Study the drawing (mm; zero at the part's minimum x, y, z) and answer. Give positions to 0.01 mm unless a question says otherwise; leave off trailing zeros. Order: outer loops, then holes, each group sorted by start corner. A loop starts at its lowest first (then second) coordinate and runs counter-clockwise, first axis right, second up. Notation, with made-up numbers: (70.5, 19) - (104.5, 19) arc R23 cw to (104.5, 35) - close; hole circle Ø8 at (11.5, 51). An arc over 180 degrees is marked (long way). Use CSV: the item, a comma, the result in double quotes.
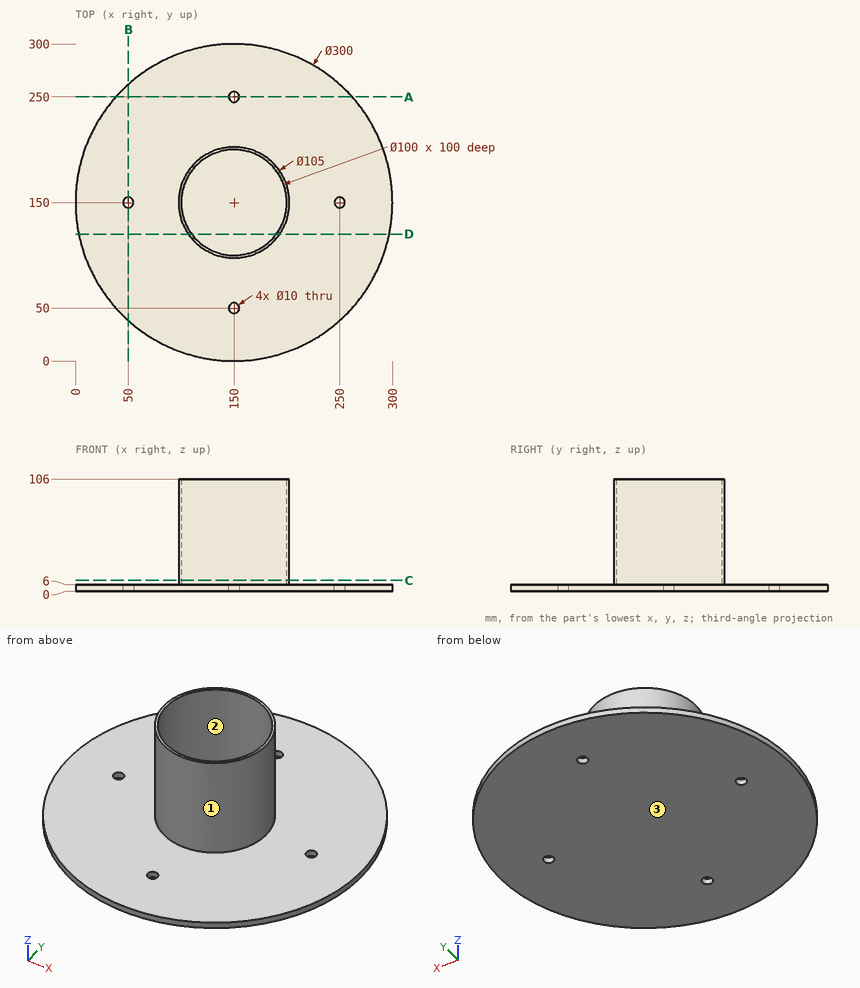
Item 1: The mould has two halves that part along Y. Classify the marked faces 1, 2 and 3: +Y half, -Y half, draft (parallel to the pull), parting line (faces both ways), or undercut.
Taken from the geometry:
face 1,"parting line"
face 2,"undercut"
face 3,"draft"
Item 2: The part is cut by section C-C (z = 10). Give the vertices of the cut face in (x, y), and give its area (3 significant figures).
Taken from the geometry:
outline,"circle Ø105 at (150, 150); hole circle Ø100 at (150, 150)"
area,"805 mm^2"
Item 3: Each of these flat-tipped pins is pushed along its axis until it touches: pin 1 (16 mm diameter, centred on x = 150, y = 250, fed in from +Z); pin 2 (1.5 mm diameter, centred on x = 113, y = 115, fed in from -Z); pin 3 (12 mm diameter, centred on x = 103, z = 32, fed in from +Y). Where does it stop, or does it pass through?
Taken from the geometry:
pin 1,"z = 6"
pin 2,"z = 0"
pin 3,"y = 182.79"
Item 4: The part is cut by section A-A (y = 250). Give the vertices of the cut face in (x, z), and give its area (3 significant figures).
Taken from the geometry:
outline,"(38.2, 0) - (145, 0) - (145, 6) - (38.2, 6) - close; (155, 0) - (261.8, 0) - (261.8, 6) - (155, 6) - close"
area,"1,280 mm^2"
Item 5: Find the intervals of material crossed by line 1 along Y through (x, z) = (150, 2.5); line 2 along Y through (x, z) = (150, 57); line 3 along Z through (x, y) = (162.5, 212), in increasing order.
Taken from the geometry:
line 1,"0 to 45, 55 to 245, 255 to 300"
line 2,"97.5 to 100, 200 to 202.5"
line 3,"0 to 6"
Item 6: The part is cut by section D-D (y = 120). Give the vertices of the cut face in (x, z), and give its area (3 significant figures).
Taken from the geometry:
outline,"(3.03, 0) - (296.97, 0) - (296.97, 6) - (193.08, 6) - (193.08, 106) - (190, 106) - (190, 6) - (110, 6) - (110, 106) - (106.92, 106) - (106.92, 6) - (3.03, 6) - close"
area,"2,380 mm^2"
